```python
from build123d import *

# Parameters (mm, degrees)
F1_DEPTH = 9.525
F3_DEPTH = 34.6458181739


# Not quite as in the source:
# - a feature names something its author has since deleted; it is built from what else it names


with BuildPart() as f1:
    # F0 (on Right) → F1 (new body)
    with BuildSketch(Plane.YZ):
        Polygon((0, 1.3819878222), (0, 0), (9.525, 0), (9.525, 35.56), (5.7011166342, 35.56), (5.7011166342, 34.6458181739), (4.7625, 34.6458181739), (3.8238833658, 34.6458181739), (3.8238833658, 35.56), (0, 35.56), (0, 33.7669878222), (0, 32.385), (0, 31.6079878222), (0, 30.226), (0, 29.4489878222), (0, 28.067), (0, 27.2899878222), (0, 25.908), (0, 25.1309878222), (0, 23.749), (0, 22.9719878222), (0, 21.59), (0, 20.8129878222), (0, 19.431), (0, 18.6539878222), (0, 17.272), (0, 16.4949878222), (0, 15.113), (0, 14.3359878222), (0, 12.954), (0, 12.1769878222), (0, 10.795), (0, 10.0179878222), (0, 8.636), (0, 7.8589878222), (0, 6.477), (0, 5.6999878222), (0, 4.318), (0, 3.5409878222), (0, 2.159), align=None)
        Polygon((-1.00000054, 0.4354505218), (0, 0), (0, 1.3819878222), (-1.00000054, 0.9465373005), (-1.00000054, 0.6909939111), align=None)
        Polygon((-1.00000054, 2.5944505218), (0, 2.159), (0, 3.5409878222), (-1.00000054, 3.1055373005), (-1.00000054, 2.8499939111), align=None)
        Polygon((-1.00000054, 4.7534505218), (0, 4.318), (0, 5.6999878222), (-1.00000054, 5.2645373005), (-1.00000054, 5.0089939111), align=None)
        Polygon((-1.00000054, 6.9124505218), (0, 6.477), (0, 7.8589878222), (-1.00000054, 7.4235373005), (-1.00000054, 7.1679939111), align=None)
        Polygon((-1.00000054, 9.0714505218), (0, 8.636), (0, 10.0179878222), (-1.00000054, 9.5825373005), (-1.00000054, 9.3269939111), align=None)
        Polygon((-1.00000054, 11.2304505218), (0, 10.795), (0, 12.1769878222), (-1.00000054, 11.7415373005), (-1.00000054, 11.4859939111), align=None)
        Polygon((-1.00000054, 13.3894505218), (0, 12.954), (0, 14.3359878222), (-1.00000054, 13.9005373005), (-1.00000054, 13.6449939111), align=None)
        Polygon((-1.00000054, 15.5484505218), (0, 15.113), (0, 16.4949878222), (-1.00000054, 16.0595373005), (-1.00000054, 15.8039939111), align=None)
        Polygon((-1.00000054, 17.7074505218), (0, 17.272), (0, 18.6539878222), (-1.00000054, 18.2185373005), (-1.00000054, 17.9629939111), align=None)
        Polygon((-1.00000054, 19.8664505218), (0, 19.431), (0, 20.8129878222), (-1.00000054, 20.3775373005), (-1.00000054, 20.1219939111), align=None)
        Polygon((0, 21.59), (0, 22.9719878222), (-1.00000054, 22.5365373005), (-1.00000054, 22.2809939111), (-1.00000054, 22.0254505218), align=None)
        Polygon((0, 23.749), (0, 25.1309878222), (-1.00000054, 24.6955373005), (-1.00000054, 24.4399939111), (-1.00000054, 24.1844505218), align=None)
        Polygon((0, 25.908), (0, 27.2899878222), (-1.00000054, 26.8545373005), (-1.00000054, 26.5989939111), (-1.00000054, 26.3434505218), align=None)
        Polygon((0, 28.067), (0, 29.4489878222), (-1.00000054, 29.0135373005), (-1.00000054, 28.7579939111), (-1.00000054, 28.5024505218), align=None)
        Polygon((0, 30.226), (0, 31.6079878222), (-1.00000054, 31.1725373005), (-1.00000054, 30.9169939111), (-1.00000054, 30.6614505218), align=None)
        Polygon((0, 32.385), (0, 33.7669878222), (-1.00000054, 33.3315373005), (-1.00000054, 33.0759939111), (-1.00000054, 32.8204505218), align=None)
    extrude(amount=F1_DEPTH)

    # F2 (on face) → F3 (cut, through all)
    with BuildSketch(Plane.XY.offset(34.6458181739)):
        with BuildLine():
            Line((4.7625, 3.96875), (4.7625, 4.7625))
            Line((4.7625, 4.7625), (3.96875, 4.7625))
            ThreePointArc((3.96875, 4.7625), (4.2012339924, 4.2012339924), (4.7625, 3.96875))
        make_face()
        with BuildLine():
            Line((3.96875, 4.7625), (4.7625, 4.7625))
            Line((4.7625, 4.7625), (4.7625, 5.55625))
            ThreePointArc((4.7625, 5.55625), (4.2012339924, 5.3237660076), (3.96875, 4.7625))
        make_face()
        with BuildLine():
            ThreePointArc((4.7625, 3.96875), (5.3237660076, 4.2012339924), (5.55625, 4.7625))
            Line((5.55625, 4.7625), (4.7625, 4.7625))
            Line((4.7625, 4.7625), (4.7625, 3.96875))
        make_face()
        with BuildLine():
            Line((4.7625, 4.7625), (5.55625, 4.7625))
            ThreePointArc((5.55625, 4.7625), (5.3237660076, 5.3237660076), (4.7625, 5.55625))
            Line((4.7625, 5.55625), (4.7625, 4.7625))
        make_face()
    extrude(amount=-F3_DEPTH, mode=Mode.SUBTRACT)


solid = f1.part
```
Geometry check sheet. Reference: the model listing, model coordinates, mm. A direction names the side the tool comes from. Coordinates: 2 decimals unless noted, no trailing zeros. Answer as a JSON object with one key per item and string values. Group by question number.
Item 1: Scan lines: probe 1 along X at (y, z) = (4.75, 12) (3 decimals); probe 2 along Y at (x, z) = (6.5, 25.5) (3 decimals); probe 3 along Z at (x, y) = (6.5, 5.25). Record each from-to range of solid material in increasing order.
Item 2: Tool access check on faces 1 (the face through (5, 5.701, 35)), 2 (the face through (5, 9.525, 18)), 3 (the face through (4.696, -0.507, 13.175)). Record the directions out of +Z, -Z, +X, -X, +Y, -Y that give a thin tool (end or side, any length) a straight path to the whole face; none if there is none.
Item 3: Depth check by flat-ended pin: pin 1 Ø4 at (x, z) = (4.5, 12) entering from -Y; pin 2 Ø0.6 at (x, z) = (5, 8) entering from -Y; pin 3 Ø0.6 at (x, z) = (5, 23) entering from -Y; pin 4 Ø0.9 at (x, z) = (7, 12.5) entering from -Y. Enter the tip coordinate at first touch or a pass-through.
Item 4: Draft check along Z on faces 4 (the face through (4.7, -0.51, 23.97)), 5 (the face through (9.525, 4, 18)), 6 (the face through (4.7, -0.51, 0.22)). Enter one of: +Z half, -Z half, draft (parallel to the pull), parting line (faces both ways), or undercut.
Resolved:
{
 "1": {"probe 1": "0 to 3.969, 5.556 to 9.525", "probe 2": "0 to 9.525", "probe 3": "0 to 34.65"},
 "2": {"face 1": "+Z, +X, -X", "face 2": "+Z, -Z, +X, -X, +Y", "face 3": "+X, -X, -Y"},
 "3": {"pin 1": "y = -1", "pin 2": "y = -0.37", "pin 3": "y = -0.62", "pin 4": "y = -0.29"},
 "4": {"face 4": "undercut", "face 5": "draft", "face 6": "-Z half"}
}
